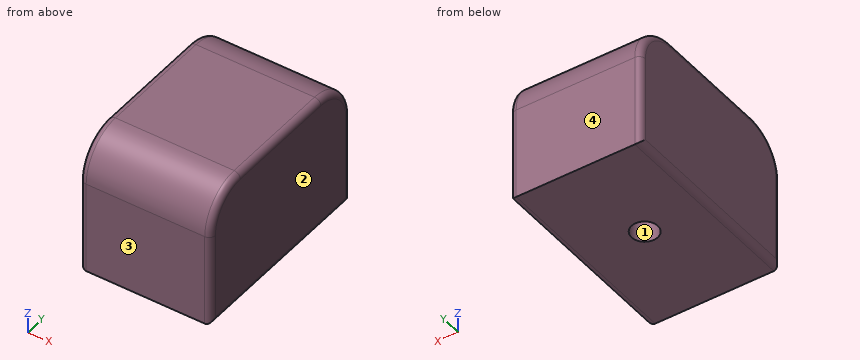
from build123d import *

# Parameters (mm, degrees)
F0_W     = 15.875
F0_H     = 24.13
F1_DEPTH = 16.256
F2_D     = 3.175
F2_DEPTH = 11.684
F2_TIP   = 0.9538662327
F3_R     = 5.08
F4_R     = 0.762


with BuildPart() as f1:
    # F0 (on Top) → F1 (new body)
    with BuildSketch(Plane.XY):
        with Locations((0.1865295499, -0.323939874)):
            Rectangle(F0_W, F0_H)
    extrude(amount=F1_DEPTH)

    # F2
    with Locations(Plane(origin=(0, 0, 0), x_dir=(1, 0, 0), z_dir=(0, 0, -1))):
        with Locations((0, 0)):
            Hole(F2_D / 2, depth=F2_DEPTH)
            with Locations((0, 0, -(F2_DEPTH + F2_TIP / 2))):  # 118° drill point
                Cone(0, F2_D / 2, F2_TIP, mode=Mode.SUBTRACT)

    # F3
    f3_edges = [f1.edges().sort_by_distance(p)[0] for p in [
        (0.18653, -12.38894, 16.256),
        (0.18653, 11.74106, 16.256),
    ]]
    fillet(f3_edges, radius=F3_R)

    # F4
    f4_edges = [f1.edges().sort_by_distance(p)[0] for p in [
        (8.12403, -12.38894, 5.588),
        (8.12403, -10.901042, 14.768102),
        (8.12403, -0.32394, 0),
        (8.12403, -0.32394, 16.256),
        (8.12403, 11.74106, 5.588),
        (8.12403, 10.253163, 14.768102),
        (-7.75097, 11.74106, 5.588),
        (-7.75097, 10.253163, 14.768102),
        (-7.75097, -0.32394, 0),
        (-7.75097, -0.32394, 16.256),
        (-7.75097, -12.38894, 5.588),
        (-7.75097, -10.901042, 14.768102),
    ]]
    fillet(f4_edges, radius=F4_R)


solid = f1.part
Build history of the part. All positions in model axes, mm. Face numbers are marked on the shaded views. Round coordinates to 2 decimals unless told otherwise and drop trailing zeros. Loops run counter-clockwise (first coordinate to the right, second up) from the corner with the lowest first, then second, coordinate; pieces in that order, holes last. Notation, with made-up numbers: (-5.5, 62) -> (10.5, 62) arc R12 cw to (10.5, 77) -> close; hole circle Ø8 at (81, 66). An arc over 180 degrees is marked (long way). One line per item, written item: value. Start each with the question number.
Q1. Probe line 1 along Y through (x, z) = (0, 3.5); line 2 along Z through (x, y) = (-5.25, 6.75); line 3 along Z through (x, y) = (-1.75, 10.75). List the from-to ranges inside material, lowest first.
Q2. Cut at B-B on x = 4.25. List the corners of the cut face in (y, z), plus the area to 3 significant figures.
Q3. Drop a flat-ended pin along its axis: pin 1 Ø8 at (x, y) = (-1, -7.5) entering from -Z. Give the stop position or say it passes through.
Q4. Cut at A-A on z = 3.5. List the corners of the cut face in (x, y) (1 decimal).
Q5. Two-plate mould, pull along Y, no slides. Class the marked faces 1, 2, 3 and 4: released by +Y, released by -Y, zero draft, split by the parting line, or undercut.
Computed:
1. line 1: -12.39 to -1.59, 1.59 to 11.74
1. line 2: 0 to 16.26
1. line 3: 0 to 14.19
2. outline: (-12.39, 0) -> (11.74, 0) -> (11.74, 11.18) arc R5.08 ccw to (6.66, 16.26) -> (-7.31, 16.26) arc R5.08 ccw to (-12.39, 11.18) -> close
2. area: 381 mm²
3. pin 1: z = 0
4. outline: (-7.8, -11.6) arc R0.8 ccw to (-7, -12.4) -> (7.4, -12.4) arc R0.8 ccw to (8.1, -11.6) -> (8.1, 11) arc R0.8 ccw to (7.4, 11.7) -> (-7, 11.7) arc R0.8 ccw to (-7.8, 11) -> close; hole circle Ø3.2 at (0, 0)
5. face 1: undercut
5. face 2: zero draft
5. face 3: released by -Y
5. face 4: released by +Y
